Check sheet for the modelled part. Datum: model origin and axes. Units: mm. A direction names the side the tool comes from. Round coordinates to 2 decimals unless told otherwise and drop trailing zeros. Write each loop counter-clockwise with the first axis right and the second up, starting at its lowest first coordinate (ties: lowest second). Pieces come first, ordered by that corner, then holes.
Item 1: Cross-section at D-D on z = 48. Enter the section's corners in (x, y), plus the area to 3 significant figures.
Item 2: Cross-section at C-C on y = 2.5. Enter the section's corners in (x, z) (3 decimals).
Item 3: Material ranges on line 1 (Z direction, x = -7.25, y = 0.5) (3 decimals); line 2 (Z direction, x = -5.25, y = 3.75) (3 decimals); line 3 (X direction, y = -0.75, z = 34.5), recorded low to high.
Item 4: Tool access check on faces 1 (the flat face through (-7.5, 1.016, -1)), 2 (the flat face through (7.5, -1.016, -1)), 3 (the cylindrical face through (-0.933, 0.294, -3.219)). Record the directions out of +Z, -Z, +X, -X, +Y, -Y that give a thin tool (end or side, any length) a straight path to the whole face; none if there is none.
Item 5: Release check for a two-part mould opening along X. For faces 4 (the cylindrical face through (-0.933, -0.294, 43.962)), 5 (the flat face through (6.985, 0, -1)), 6 (the flat face through (0, 7.747, 17)) record: +X half, -X half, draft (parallel to the pull), parting line (faces both ways), or undercut.
Item 6: Go/stop test with flat-tipped pins: pin 1 Ø0.5 at (x, y) = (-7.5, 0.5) entering from -Z; pin 2 Ø4.5 at (x, y) = (-4, 0) entering from -Z; pin 3 Ø1.5 at (y, z) = (2.5, 35) entering from +X. Record where each tip stops, or that it passes through.
Item 7: Cross-section at A-A on x = 0. Enter the section's corners in (y, z) (3 decimals).
Item 8: Cross-section at B-B on z = 12. Enter the section's corners in (x, y) (3 decimals).
from build123d import *

# Parameters (mm, degrees)
BOSS_EXTRUDE1_DEPTH = 34.925
SKETCH2_R           = 3.175
BOSS_EXTRUDE2_DEPTH = 1.524
SKETCH3_R           = 0.9779
BOSS_EXTRUDE3_DEPTH = 15.24
BOSS_EXTRUDE4_START = 6.35
SKETCH4_R           = 0.9779
BOSS_EXTRUDE4_DEPTH = 6.35
SKETCH5_W           = 1.016
SKETCH5_H           = 2.032
BOSS_EXTRUDE5_DEPTH = 2.032


with BuildPart() as part:
    # Sketch1 → Boss-Extrude1 (new body)
    with BuildSketch(Plane.XY):
        with BuildLine():
            Line((7.517713482, 7.747), (-7.517713482, 7.747))
            ThreePointArc((-7.517713482, 7.747), (-10.795, 0), (-7.517713482, -7.747))
            Line((-7.517713482, -7.747), (7.517713482, -7.747))
            ThreePointArc((7.517713482, -7.747), (9.941975207, -4.205847594), (10.795, 0))
            ThreePointArc((10.795, 0), (9.941975207, 4.205847594), (7.517713482, 7.747))
        make_face()
    extrude(amount=BOSS_EXTRUDE1_DEPTH)

    # Sketch2 → Boss-Extrude2 (add)
    with BuildSketch(Plane.XY.offset(34.925)):
        with Locations(Location((0, 0, 0), (0, 0, 180))):
            Circle(SKETCH2_R)
    extrude(amount=BOSS_EXTRUDE2_DEPTH)

    # Sketch3 → Boss-Extrude3 (add)
    with BuildSketch(Plane.XY.offset(36.449)):
        with Locations(Location((0, 0, 0), (0, 0, 180))):
            Circle(SKETCH3_R)
    extrude(amount=BOSS_EXTRUDE3_DEPTH)

    # Sketch4 → Boss-Extrude4 (add)
    with BuildSketch(Plane(origin=(0, 0, 0), x_dir=(-1, 0, 0), z_dir=(0, 0, -1)).offset(BOSS_EXTRUDE4_START)):
        Circle(SKETCH4_R)
    extrude(amount=-BOSS_EXTRUDE4_DEPTH)

    # Sketch5 → Boss-Extrude5 (add)
    with BuildSketch(Plane(origin=(0, 0, 0), x_dir=(-1, 0, 0), z_dir=(0, 0, -1))):
        with Locations((-7.493, 0)):
            Rectangle(SKETCH5_W, SKETCH5_H)
        with Locations((7.493, 0)):
            Rectangle(SKETCH5_W, SKETCH5_H)
    extrude(amount=BOSS_EXTRUDE5_DEPTH)


solid = part.part
Response values:
1. outline: circle Ø1.96 at (0, 0)
1. area: 3.00 mm2
2. outline: (-10.502, 0) - (10.502, 0) - (10.502, 34.925) - (1.957, 34.925) - (1.957, 36.449) - (-1.957, 36.449) - (-1.957, 34.925) - (-10.502, 34.925) - close
3. line 1: z = -2.032 to 34.925
3. line 2: z = 0 to 34.925
3. line 3: x = -10.77 to 10.77
4. face 1: -Z, +X, -X, +Y
4. face 2: -Z, +X, -X, -Y
4. face 3: -Z
5. face 4: parting line
5. face 5: undercut
5. face 6: draft
6. pin 1: stops at z = -2.03
6. pin 2: stops at z = 0
6. pin 3: stops at x = 10.65
7. outline: (-7.747, 0) - (-0.978, 0) - (-0.978, -6.35) - (0.978, -6.35) - (0.978, 0) - (7.747, 0) - (7.747, 34.925) - (3.175, 34.925) - (3.175, 36.449) - (0.978, 36.449) - (0.978, 51.689) - (-0.978, 51.689) - (-0.978, 36.449) - (-3.175, 36.449) - (-3.175, 34.925) - (-7.747, 34.925) - close
8. outline: (-7.518, -7.747) - (7.518, -7.747) arc R10.795 ccw to (7.518, 7.747) - (-7.518, 7.747) arc R10.795 ccw to start
